```python
from build123d import *

# Parameters (mm, degrees)
SKETCH1_W           = 23
SKETCH1_H           = 17
BOSS_EXTRUDE1_DEPTH = 2.5
SKETCH2_W           = 13
SKETCH2_H           = 6
BOSS_EXTRUDE2_DEPTH = 18
SKETCH3_W           = 23
SKETCH3_H           = 17
BOSS_EXTRUDE3_DEPTH = 2.5
SKETCH5_W           = 2
SKETCH5_H           = 3
CUT_EXTRUDE1_DEPTH  = 24
SKETCH4_R           = 1.25
CUT_EXTRUDE3_DEPTH  = 24
SKETCH7_R           = 1.25
CUT_EXTRUDE4_DEPTH  = 10


with BuildPart() as part:
    # Sketch1 → Boss-Extrude1 (new body)
    with BuildSketch(Plane(origin=(0, 0, 0), x_dir=(0, 0, -1), z_dir=(1, 0, 0))):
        with Locations((-39.471099191, 23.847043717)):
            Rectangle(SKETCH1_W, SKETCH1_H)
    extrude(amount=BOSS_EXTRUDE1_DEPTH)

    # Sketch2 → Boss-Extrude2 (add)
    with BuildSketch(Plane(origin=(2.5, 0, 0), x_dir=(0, 0, -1), z_dir=(1, 0, 0))):
        with Locations((-34.471099191, 18.347043717)):
            Rectangle(SKETCH2_W, SKETCH2_H)
    extrude(amount=BOSS_EXTRUDE2_DEPTH)

    # Sketch3 → Boss-Extrude3 (add)
    with BuildSketch(Plane(origin=(20.5, 0, 0), x_dir=(0, 0, -1), z_dir=(1, 0, 0))):
        with Locations((-39.471099191, 23.847043717)):
            Rectangle(SKETCH3_W, SKETCH3_H)
    extrude(amount=BOSS_EXTRUDE3_DEPTH)

    # Sketch5 → Cut-Extrude1 (cut, through all)
    with BuildSketch(Plane(origin=(23, 0, 0), x_dir=(0, 0, -1), z_dir=(1, 0, 0))):
        with Locations((-49.971099191, 16.847043717)):
            Rectangle(SKETCH5_W, SKETCH5_H)
    extrude(amount=-CUT_EXTRUDE1_DEPTH, mode=Mode.SUBTRACT)

    # Sketch4 → Cut-Extrude3 (cut, through all)
    with BuildSketch(Plane(origin=(23, 0, 0), x_dir=(0, 0, -1), z_dir=(1, 0, 0))):
        with Locations((-47.611099191, 28.347043717)):
            Circle(SKETCH4_R)
    extrude(amount=-CUT_EXTRUDE3_DEPTH, mode=Mode.SUBTRACT)

    # Sketch7 → Cut-Extrude4 (cut)
    with BuildSketch(Plane(origin=(0, 21.347043717, 0), x_dir=(1, 0, 0), z_dir=(0, 1, 0))):
        with Locations((7.5, -32.971099191)):
            Circle(SKETCH7_R)
        with Locations((15.5, -32.971099191)):
            Circle(SKETCH7_R)
    extrude(amount=-CUT_EXTRUDE4_DEPTH, mode=Mode.SUBTRACT)


solid = part.part
```
CAD build for the part. Positions are in the model's coordinates, mm. A direction names the side the tool comes from. Coordinates: 2 decimals unless noted, no trailing zeros. Loops run counter-clockwise (first coordinate to the right, second up) from the corner with the lowest first, then second, coordinate; pieces in that order, holes last. Notation, with made-up numbers: (-13, -11) - (20, -11) arc R31 ccw to (20, 17) - close; hole circle Ø1 at (-5, -33). An arc over 180 degrees is marked (long way). Use CSV: the item, a comma, the result in double quotes. Start each with the question number.
Q1. Cut at C-C, the plane z = 48.5. List the corners of the cut face in (x, y), then the cut area to 3 significant figures.
Q2. Cut at A-A, the plane x = 7.5. List the corners of the cut face in (y, z).
Q3. 3-axis set-ups, long thin cutter, end or side, ignore diameter. For faces 5 (the flat face through (1, 32.347, 40)), 6 (the cylindrical face through (7.23, 18.39, 34.19)), 7 (the flat face through (22, 18.347, 50)), 8 (the flat face through (20.5, 26, 40)), 9 (the flat face through (11, 18, 40.971)): which of +Z, -Z, +X, -X, +Y, -Y reach the whole face in a straight line?
Q4. Drop flat-ended pins along their axis: P1, Ø8.5, axis at y = 28, z = 35, coming from the -X side; P2, Ø0.8, axis at x = 21.5, y = 16.5, coming from the +Z side; P3, Ø3, axis at x = 13.5, y = 19, coming from the +Z side; P4, Ø1.6, axis at x = 21.5, z = 50, coming from the -Y side. Give the stop position or say it passes through.
Q5. Cut at B-B, the plane z = 43.25. List the corners of the cut face in (x, y).
Q6. Cut at D-D, the plane z = 40. List the corners of the cut face in (x, y).
Q7. Probe probe 1 along X at (y, z) = (28, 38.5); probe 2 along Z at (x, y) = (7.5, 18.4); probe 3 along Y at (x, z) = (14, 39.25). List the from-to ranges inside material, lowest first. Write a range as from..to.
Q8. Two-plate mould, pull along X, no slides. Class faces 1 (the flat face through (22, 25, 50.971)), 2 (the flat face through (2.5, 26, 40)), 3 (the flat face through (23, 24, 40)), 4 (the flat face through (11, 21.347, 35)): +X half, -X half, draft (parallel to the pull), parting line (faces both ways), or undercut.
Here are the results:
1,outline,"(0, 15.35) - (2.5, 15.35) - (2.5, 27.47) - (0, 27.47) - close; (0, 29.23) - (2.5, 29.23) - (2.5, 32.35) - (0, 32.35) - close; (20.5, 15.35) - (23, 15.35) - (23, 27.47) - (20.5, 27.47) - close; (20.5, 29.23) - (23, 29.23) - (23, 32.35) - (20.5, 32.35) - close"
1,area,"76.2 mm2"
2,outline,"(15.35, 27.97) - (21.35, 27.97) - (21.35, 31.72) - (15.35, 31.72) - close; (15.35, 34.22) - (21.35, 34.22) - (21.35, 40.97) - (15.35, 40.97) - close"
3,face 5,"+Z, -Z, +X, -X, +Y"
3,face 6,"+Y, -Y"
3,face 7,"+Z, +X, -X, -Y"
3,face 8,"+Z, +Y"
3,face 9,"+Z, +Y, -Y"
4,P1,"x = 0"
4,P2,"z = 48.97"
4,P3,"z = 40.97"
4,P4,"y = 18.35"
5,outline,"(0, 15.35) - (2.5, 15.35) - (2.5, 32.35) - (0, 32.35) - close; (20.5, 15.35) - (23, 15.35) - (23, 32.35) - (20.5, 32.35) - close"
6,outline,"(0, 15.35) - (23, 15.35) - (23, 32.35) - (20.5, 32.35) - (20.5, 21.35) - (2.5, 21.35) - (2.5, 32.35) - (0, 32.35) - close"
7,probe 1,"0..2.5, 20.5..23"
7,probe 2,"27.97..31.72, 34.22..40.97"
7,probe 3,"15.35..21.35"
8,face 1,"draft"
8,face 2,"undercut"
8,face 3,"+X half"
8,face 4,"undercut"
